```python
from build123d import *

# Parameters (mm, degrees)
SKETCH1_W           = 65
SKETCH1_H           = 115
SKETCH1_W_2         = 55
SKETCH1_H_2         = 105
BOSS_EXTRUDE1_DEPTH = 23
FILLET1_R           = 6
SKETCH2_R           = 6
BOSS_EXTRUDE2_DEPTH = 23
SKETCH4_R           = 2.2
CUT_EXTRUDE1_DEPTH  = 23
SKETCH7_W           = 55
SKETCH7_H           = 105
CUT_EXTRUDE2_DEPTH  = 13
SKETCH8_W           = 65
SKETCH8_H           = 11.5
CUT_EXTRUDE3_DEPTH  = 120
SKETCH9_R           = 5
CUT_EXTRUDE4_DEPTH  = 6.5
BOSS_EXTRUDE3_DEPTH = 11.5


with BuildPart() as part:
    # Sketch1 → Boss-Extrude1 (new body)
    with BuildSketch(Plane(origin=(0, 0, 0), x_dir=(1, 0, 0), z_dir=(0, 1, 0))):
        Rectangle(SKETCH1_W, SKETCH1_H)
        Rectangle(SKETCH1_W_2, SKETCH1_H_2, mode=Mode.SUBTRACT)
    extrude(amount=BOSS_EXTRUDE1_DEPTH)

    # Fillet1
    fillet1_edges = [part.edges().sort_by_distance(p)[0] for p in [
        (32.5, 11.5, 57.5),
        (-32.5, 11.5, 57.5),
        (-32.5, 11.5, -57.5),
        (32.5, 11.5, -57.5),
    ]]
    fillet(fillet1_edges, radius=FILLET1_R)

    # Sketch2 → Boss-Extrude2 (add)
    with BuildSketch(Plane(origin=(0, 23, 0), x_dir=(1, 0, 0), z_dir=(0, 1, 0))):
        with Locations((-26.5, 51.5)):
            Circle(SKETCH2_R)
        with Locations((26.5, 51.5)):
            Circle(SKETCH2_R)
        with Locations((-26.5, -51.5)):
            Circle(SKETCH2_R)
        with Locations((26.5, -51.5)):
            Circle(SKETCH2_R)
    extrude(amount=-BOSS_EXTRUDE2_DEPTH)

    # Sketch4 → Cut-Extrude1 (cut)
    with BuildSketch(Plane(origin=(0, 23, 0), x_dir=(1, 0, 0), z_dir=(0, 1, 0))):
        with Locations(Location((-26.5, 51.5, 0), (0, 0, 270))):
            Circle(SKETCH4_R)
        with Locations(Location((26.5, 51.5, 0), (0, 0, 270))):
            Circle(SKETCH4_R)
        with Locations(Location((26.5, -51.5, 0), (0, 0, 270))):
            Circle(SKETCH4_R)
        with Locations(Location((-26.5, -51.5, 0), (0, 0, 270))):
            Circle(SKETCH4_R)
    extrude(amount=-CUT_EXTRUDE1_DEPTH, mode=Mode.SUBTRACT)

    # Sketch7 → Cut-Extrude2 (cut)
    with BuildSketch(Plane(origin=(0, 18, 0), x_dir=(1, 0, 0), z_dir=(0, 1, 0))):
        Rectangle(SKETCH7_W, SKETCH7_H)
    extrude(amount=-CUT_EXTRUDE2_DEPTH, mode=Mode.SUBTRACT)

    # Sketch8 → Cut-Extrude3 (cut)
    with BuildSketch(Plane.XY.offset(57.5)):
        with Locations((0, 5.75)):
            Rectangle(SKETCH8_W, SKETCH8_H)
    extrude(amount=-CUT_EXTRUDE3_DEPTH, mode=Mode.SUBTRACT)

    # Sketch9 → Cut-Extrude4 (cut)
    with BuildSketch(Plane.XZ.offset(-18)):
        with Locations((-26.5, -51.5)):
            Circle(SKETCH9_R)
        with Locations((26.5, -51.5)):
            Circle(SKETCH9_R)
        with Locations((26.5, 51.5)):
            Circle(SKETCH9_R)
        with Locations((-26.5, 51.5)):
            Circle(SKETCH9_R)
    extrude(amount=CUT_EXTRUDE4_DEPTH, mode=Mode.SUBTRACT)

    # Sketch10 → Boss-Extrude3 (add)
    with BuildSketch(Plane(origin=(0, 23, 0), x_dir=(1, 0, 0), z_dir=(0, 1, 0))):
        with BuildLine():
            Line((-26.5, -59.5), (26.5, -59.5))
            ThreePointArc((26.5, -59.5), (32.156854249, -57.156854249), (34.5, -51.5))
            Line((34.5, -51.5), (34.5, 51.5))
            ThreePointArc((34.5, 51.5), (32.156854249, 57.156854249), (26.5, 59.5))
            Line((26.5, 59.5), (-26.5, 59.5))
            ThreePointArc((-26.5, 59.5), (-32.156854249, 57.156854249), (-34.5, 51.5))
            Line((-34.5, 51.5), (-34.5, -51.5))
            ThreePointArc((-34.5, -51.5), (-32.156854249, -57.156854249), (-26.5, -59.5))
        make_face()
        with BuildLine():
            Line((-26.5, -57.5), (26.5, -57.5))
            ThreePointArc((26.5, -57.5), (30.742640687, -55.742640687), (32.5, -51.5))
            Line((32.5, -51.5), (32.5, 51.5))
            ThreePointArc((32.5, 51.5), (30.742640687, 55.742640687), (26.5, 57.5))
            Line((26.5, 57.5), (-26.5, 57.5))
            ThreePointArc((-26.5, 57.5), (-30.742640687, 55.742640687), (-32.5, 51.5))
            Line((-32.5, 51.5), (-32.5, -51.5))
            ThreePointArc((-32.5, -51.5), (-30.742640687, -55.742640687), (-26.5, -57.5))
        make_face(mode=Mode.SUBTRACT)
    extrude(amount=-BOSS_EXTRUDE3_DEPTH)


solid = part.part
```
Verification items for the finished model (mm, model axes). A direction names the side the tool comes from. Give positions to 0.01 mm unless a question says otherwise; leave off trailing zeros. Loops run counter-clockwise (first coordinate to the right, second up) from the corner with the lowest first, then second, coordinate; pieces in that order, holes last. Notation, with made-up numbers: M 7.5,72 L 46.5,72 A22 cw 46.5,107 Z; hole C 4,12.25 d9. An arc over 180 degrees is marked long. Return JSON: item names as keys, results as strings.
1) Gauge pin test, flat ends, axial feed: P1, Ø3.5, axis at x = -26.5, z = 51.5, coming from the +Y side; P2, Ø8, axis at x = -26.5, z = -51.5, coming from the -Y side. Record the tip position at first contact, or that the pin passes through.
Findings:
{"P1": "passes through", "P2": "stops at y = 18"}
2) Material ranges on L1, parallel to X at y = 18.25, z = 0.5; L2, parallel to X at y = 21.45, z = 51.5; L3, parallel to Z at x = 13, y = 12.25, recorded low to high. Write a range as [from, to].
Findings:
{"L1": "x = [-34.5, -27.5], [27.5, 34.5]", "L2": "x = [-34.5, -28.7], [-24.3, -20.5], [20.5, 24.3], [28.7, 34.5]", "L3": "z = [-59.5, -52.5], [52.5, 59.5]"}
3) Section check D-D, the plane y = 21.5. Enter the section's corners in (x, z), and give its area (3 significant figures).
Findings:
{"outline": "M -34.5,-51.5 A8 ccw -26.5,-59.5 L 26.5,-59.5 A8 ccw 34.5,-51.5 L 34.5,51.5 A8 ccw 26.5,59.5 L -26.5,59.5 A8 ccw -34.5,51.5 Z; hole C -26.5,-51.5 d4.4; hole C -26.5,51.5 d4.4; hole M -27.5,-45.58 A6 cw -20.58,-52.5 L 20.58,-52.5 A6 cw 27.5,-45.58 L 27.5,45.58 A6 cw 20.58,52.5 L -20.58,52.5 A6 cw -27.5,45.58 Z; hole C 26.5,-51.5 d4.4; hole C 26.5,51.5 d4.4", "area": "2,490 mm2"}
4) Section check C-C, the plane y = 15. Enter the section's corners in (x, z), and give its area (3 significant figures).
Findings:
{"outline": "M -34.5,-51.5 A8 ccw -26.5,-59.5 L 26.5,-59.5 A8 ccw 34.5,-51.5 L 34.5,51.5 A8 ccw 26.5,59.5 L -26.5,59.5 A8 ccw -34.5,51.5 Z; hole M -27.5,-46.6 A5 ccw long -21.6,-52.5 L 21.6,-52.5 A5 ccw long 27.5,-46.6 L 27.5,46.6 A5 ccw long 21.6,52.5 L -21.6,52.5 A5 ccw long -27.5,46.6 Z", "area": "2,190 mm2"}
5) Mould release check, pull along X, two halves, no side actions. Record for faces 3 (the cylindrical face through (-27.839, 20.535, -53.246)), 4 (the flat face through (-28, 11.5, 0)): released by +X, released by -X, zero draft, split by the parting line, or undercut.
Findings:
{"face 3": "undercut", "face 4": "zero draft"}
6) Section check B-B, the plane z = 25. Enter the section's corners in (x, y).
Findings:
{"outline": "M -34.5,11.5 L -27.5,11.5 L -27.5,23 L -34.5,23 Z; M 27.5,11.5 L 34.5,11.5 L 34.5,23 L 27.5,23 Z"}
7) Section check A-A, the plane x = -13. Enter the section's corners in (y, z), and give its area (3 significant figures).
Findings:
{"outline": "M 11.5,-59.5 L 23,-59.5 L 23,-52.5 L 11.5,-52.5 Z; M 11.5,52.5 L 23,52.5 L 23,59.5 L 11.5,59.5 Z", "area": "161 mm2"}
8) Tool access check on faces 1 (the cylindrical face through (-29.93, 14.8, 55.14)), 2 (the cylindrical face through (25.161, 20.535, -53.246)). Record the directions out of +Z, -Z, +X, -X, +Y, -Y that give a thin tool (end or side, any length) a straight path to the whole face; none if there is none.
Findings:
{"face 1": "-Y", "face 2": "+Y, -Y"}
